Part model, mm, in its own coordinate system. Face numbers are marked on the shaded views. Coordinates: 2 decimals unless noted, no trailing zeros. Loops run counter-clockwise (first coordinate to the right, second up) from the corner with the lowest first, then second, coordinate; pieces in that order, holes last. Notation, with made-up numbers: (-21.5, 75.5) -> (-16.5, 75.5) arc R15 cw to (-16.5, 94.5) -> close; hole circle Ø9 at (25.5, 41). An arc over 180 degrees is marked (long way). One line per question, with ' | ' between items. Start each with the question number.
1) Cut at A-A (z = -1.2). List the corners of the cut face in (x, y).
2) Probe L1, parallel to X at y = -1.5, z = 1.9; L2, parallel to Y at x = 32, z = -0.1. List the from-to ranges inside material, lowest first. Write a range as from..to.
3) Two-plate mould, pull along Z, no slides. Class the marked faces 1 and 2: released by +Z, released by -Z, zero draft, split by the parting line, or undercut.
from build123d import *

# Parameters (mm, degrees)
SKETCH1_W           = 150
SKETCH1_H           = 70
BOSS_EXTRUDE1_DEPTH = 2.5
SKETCH2_R           = 4
CUT_EXTRUDE1_DEPTH  = 6
SKETCH3_W           = 30
SKETCH3_H           = 70
CUT_EXTRUDE2_DEPTH  = 6


with BuildPart() as part:
    # Sketch1 → Boss-Extrude1 (new body, symmetric)
    with BuildSketch(Plane.XY):
        Rectangle(SKETCH1_W, SKETCH1_H)
    extrude(amount=BOSS_EXTRUDE1_DEPTH, both=True)

    # Sketch2 → Cut-Extrude1 (cut, through all)
    with BuildSketch(Plane.XY.offset(2.5)):
        with Locations((63, 0.628549325)):
            Circle(SKETCH2_R)
        with Locations((29.001496193, 0.309583996)):
            Circle(SKETCH2_R)
        with Locations((-42.995335398, -0.365871995)):
            Circle(SKETCH2_R)
        with Locations((-3.99705162, 0)):
            Circle(SKETCH2_R)
    extrude(amount=-CUT_EXTRUDE1_DEPTH, mode=Mode.SUBTRACT)

    # Sketch3 → Cut-Extrude2 (cut, through all)
    with BuildSketch(Plane.XY.offset(2.5)):
        with Locations((60, 0)):
            Rectangle(SKETCH3_W, SKETCH3_H)
    extrude(amount=-CUT_EXTRUDE2_DEPTH, mode=Mode.SUBTRACT)


solid = part.part
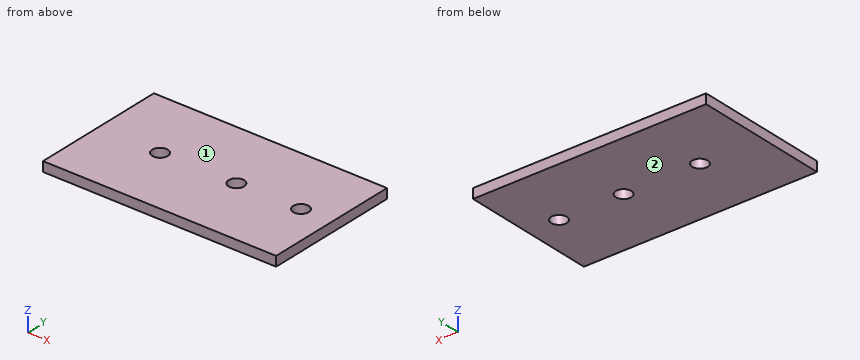
Reported:
1) outline: (-75, -35) -> (45, -35) -> (45, 35) -> (-75, 35) -> close; hole circle Ø8 at (-43, -0.37); hole circle Ø8 at (-4, 0); hole circle Ø8 at (29, 0.31)
2) L1: x = -75..-46.83, -39.16..-7.71, -0.29..25.43, 32.57..45 | L2: y = -35..-2.34, 2.96..35
3) face 1: released by +Z | face 2: released by -Z
